Check sheet for the modelled part. Datum: model origin and axes. Units: mm. A direction names the side the tool comes from. Round coordinates to 2 decimals unless told otherwise and drop trailing zeros. Loops run counter-clockwise (first coordinate to the right, second up) from the corner with the lowest first, then second, coordinate; pieces in that order, holes last. Notation, with made-up numbers: (-35.5, 48) - (-23.5, 48) arc R9 cw to (-23.5, 64) - close; hole circle Ø2 at (52, 57). An arc over 180 degrees is marked (long way). Put each result on its own line as item: value.
```python
from build123d import *

# Parameters (mm, degrees)
BOSS_EXTRUDE1_DEPTH = 10
SKETCH2_W           = 5
SKETCH2_H           = 32
BOSS_EXTRUDE2_DEPTH = 18
SKETCH3_W           = 24
SKETCH3_H           = 20
BOSS_EXTRUDE3_DEPTH = 7
CUT_EXTRUDE1_DEPTH  = 56.290143787
BOSS_EXTRUDE4_REACH = 56.194
SKETCH7_R           = 1.7
CUT_EXTRUDE2_DEPTH  = 7
SKETCH6_W           = 8
SKETCH6_H           = 2.8
CUT_EXTRUDE3_DEPTH  = 13.34
SKETCH8_R           = 1.95
CUT_EXTRUDE4_DEPTH  = 55.194244669
FILLET1_R           = 5
FILLET2_R           = 1.25
FILLET3_R           = 6
SKETCH9_W           = 18
SKETCH9_H           = 2.5
BOSS_EXTRUDE5_DEPTH = 4
FILLET4_R           = 1


with BuildPart() as part:
    # Sketch1 → Boss-Extrude1 (new body)
    with BuildSketch(Plane(origin=(0, 0, 0), x_dir=(1, 0, 0), z_dir=(0, 1, 0))):
        Polygon((-17.769938204, -26), (-17.769938204, -20), (-7.769938204, -20), (-7.769938204, 0), (-17.769938204, 0), (-17.769938204, 6), (26.230061796, 6), (26.230061796, 0), (16.230061796, 0), (16.230061796, -20), (26.230061796, -20), (26.230061796, -26), align=None)
    extrude(amount=BOSS_EXTRUDE1_DEPTH)

    # Sketch2 → Boss-Extrude2 (add)
    with BuildSketch(Plane(origin=(0, 10, 0), x_dir=(1, 0, 0), z_dir=(0, 1, 0))):
        with Locations((-5.269938204, -10)):
            Rectangle(SKETCH2_W, SKETCH2_H)
        with Locations((13.730061796, -10)):
            Rectangle(SKETCH2_W, SKETCH2_H)
    extrude(amount=BOSS_EXTRUDE2_DEPTH)

    # Sketch3 → Boss-Extrude3 (add)
    with BuildSketch(Plane(origin=(0, 28, 0), x_dir=(1, 0, 0), z_dir=(0, 1, 0))):
        with Locations((4.230061796, -10)):
            Rectangle(SKETCH3_W, SKETCH3_H)
    extrude(amount=BOSS_EXTRUDE3_DEPTH)

    # Sketch4 → Cut-Extrude1 (cut, through all)
    with BuildSketch(Plane(origin=(16.230061796, 0, 0), x_dir=(0, 0, -1), z_dir=(1, 0, 0))):
        with BuildLine():
            Line((-26, 10), (-26, 35))
            Line((-26, 35), (-18.555107994, 35))
            add(Edge.make_bspline(
                [(-26, 10), (-25.555357091, 18.878891188), (-18.529592831, 25.955762579), (-18.555107994, 35)],
                knots=[0, 0, 0, 0, 1, 1, 1, 1], degree=3))
        make_face()
        with BuildLine():
            Line((6, 10), (6, 35))
            Line((6, 35), (-1.444892006, 35))
            add(Edge.make_bspline(
                [(6, 10), (5.555357091, 18.878891188), (-1.470407169, 25.955762579), (-1.444892006, 35)],
                knots=[0, 0, 0, 0, 1, 1, 1, 1], degree=3))
        make_face()
    extrude(amount=-CUT_EXTRUDE1_DEPTH, mode=Mode.SUBTRACT)

    # Boss-Extrude4: up to this face of the body (flat: up to its plane)
    boss_extrude4_end = Plane(part.part.faces().sort_by_distance((4.230061796, 5, -6))[0])
    # Sketch5 → Boss-Extrude4 (add, up to the picked face)
    with BuildSketch(Plane.XY.offset(26), mode=Mode.PRIVATE) as boss_extrude4_sk1:
        with BuildLine():
            Line((-2.769938204, 10), (11.230061796, 10))
            Line((11.230061796, 10), (11.230061796, 16.5))
            ThreePointArc((11.230061796, 16.5), (11.083615187, 16.853553391), (10.730061796, 17))
            Line((10.730061796, 17), (9.730061796, 17))
            Line((9.730061796, 17), (4.598638866, 11.402084076))
            ThreePointArc((4.598638866, 11.402084076), (4.230061796, 11.239946391), (3.861484726, 11.402084076))
            Line((3.861484726, 11.402084076), (-1.269938204, 17))
            Line((-1.269938204, 17), (-2.269938204, 17))
            ThreePointArc((-2.269938204, 17), (-2.623491594, 16.853553391), (-2.769938204, 16.5))
            Line((-2.769938204, 16.5), (-2.769938204, 10))
        make_face()
    boss_extrude4_tool1 = split(extrude(boss_extrude4_sk1.sketch, amount=-BOSS_EXTRUDE4_REACH, mode=Mode.PRIVATE), bisect_by=boss_extrude4_end, keep=Keep.BOTH, mode=Mode.PRIVATE)
    add(boss_extrude4_tool1.solids().sort_by(Axis((-2.613413, 13.25, 26), (0, 0, -1)))[0])

    # Sketch7 → Cut-Extrude2 (cut)
    with BuildSketch(Plane(origin=(0, 35, 0), x_dir=(1, 0, 0), z_dir=(0, 1, 0))):
        with Locations(Location((4.230061796, -10.360107994, 0), (0, 0, 270))):
            Circle(SKETCH7_R)
    extrude(amount=-CUT_EXTRUDE2_DEPTH, mode=Mode.SUBTRACT)

    # Sketch6 → Cut-Extrude3 (cut)
    with BuildSketch(Plane.XY.offset(20.5)):
        with Locations((4.230061796, 31.5)):
            Rectangle(SKETCH6_W, SKETCH6_H)
    extrude(amount=-CUT_EXTRUDE3_DEPTH, mode=Mode.SUBTRACT)

    # Sketch8 → Cut-Extrude4 (cut, through all)
    with BuildSketch(Plane.XY.offset(26)):
        with Locations((21.230061796, 5)):
            Circle(SKETCH8_R)
        with Locations((-12.769938204, 5)):
            Circle(SKETCH8_R)
    extrude(amount=-CUT_EXTRUDE4_DEPTH, mode=Mode.SUBTRACT)

    # Fillet1
    fillet1_edges = [part.edges().sort_by_distance(p)[0] for p in [
        (-17.769938204, 0, -3),
        (-17.769938204, 10, -3),
        (-17.769938204, 0, 23),
        (-17.769938204, 10, 23),
        (26.230061796, 10, -3),
        (26.230061796, 0, -3),
        (26.230061796, 0, 23),
        (26.230061796, 10, 23),
    ]]
    fillet(fillet1_edges, radius=FILLET1_R - 0.0001)  # a hair under: the kernel refuses the full size

    # Fillet2
    fillet2_edges = [part.edges().sort_by_distance(p)[0] for p in [
        (-7.769938204, 5, 20),
        (-7.769938204, 5, 0),
        (16.230061796, 5, 0),
        (16.230061796, 5, 20),
    ]]
    fillet(fillet2_edges, radius=FILLET2_R)

    # Fillet3
    fillet3_edges = [part.edges().sort_by_distance(p)[0] for p in [
        (16.230061796, 35, 10),
        (-7.769938204, 35, 10),
    ]]
    fillet(fillet3_edges, radius=FILLET3_R)

    # Sketch9 → Boss-Extrude5 (add)
    with BuildSketch(Plane.XZ):
        with Locations((4.230061796, 24.75)):
            Rectangle(SKETCH9_W, SKETCH9_H)
    extrude(amount=BOSS_EXTRUDE5_DEPTH)

    # Fillet4
    fillet4_edges = [part.edges().sort_by_distance(p)[0] for p in [
        (4.230061796, 0, 23.5),
    ]]
    fillet(fillet4_edges, radius=FILLET4_R)


solid = part.part
```
Item 1: Section check C-C on y = 8.5. Enter the section's corners in (x, z), then the cut area to 3 significant figures.
Filled sheet:
outline: (-16.34, -6) - (24.8, -6) - (24.8, 0) - (17.48, 0) arc R1.25 cw to (16.23, 1.25) - (16.23, 18.75) arc R1.25 cw to (17.48, 20) - (24.8, 20) - (24.8, 26) - (-16.34, 26) - (-16.34, 20) - (-9.02, 20) arc R1.25 cw to (-7.77, 18.75) - (-7.77, 1.25) arc R1.25 cw to (-9.02, 0) - (-16.34, 0) - close
area: 975 mm²
Item 2: Section check A-A on z = 14.5. Enter the section's corners in (x, y), then the cut area to 3 significant figures.
Filled sheet:
outline: (-7.77, 0) - (16.23, 0) - (16.23, 29) arc R6 ccw to (10.23, 35) - (-1.77, 35) arc R6 ccw to (-7.77, 29) - close; hole (-2.77, 16.5) arc R0.5 cw to (-2.27, 17) - (-1.27, 17) - (3.86, 11.4) arc R0.5 ccw to (4.6, 11.4) - (9.73, 17) - (10.73, 17) arc R0.5 cw to (11.23, 16.5) - (11.23, 28) - (-2.77, 28) - close; hole (0.23, 30.1) - (8.23, 30.1) - (8.23, 32.9) - (0.23, 32.9) - close
area: 615 mm²
Item 3: Release check for a two-part mould opening along Z. For faces 6 (the flat face through (19, 10, -3)), 7 (the flat face through (22, 3, 0)), 8 (the flat face through (4, 6, -6)) record: +Z half, -Z half, draft (parallel to the pull), parting line (faces both ways), or undercut.
Filled sheet:
face 6: draft
face 7: undercut
face 8: -Z half
Item 4: Section check B-B on x = -12. Enter the section's corners in (y, z).
Filled sheet:
outline: (0, -6) - (3.21, -6) - (3.21, 0) - (0, 0) - close; (0, 20) - (3.21, 20) - (3.21, 26) - (0, 26) - close; (6.79, -6) - (10, -6) - (10, 0) - (6.79, 0) - close; (6.79, 20) - (10, 20) - (10, 26) - (6.79, 26) - close
Item 5: Thickness scan on line 1 (Z direction, x = 19, y = 5); line 2 (Y direction, x = 3, z = 17.5); line 3 (Y direction, x = 8, z = 8.5). Record the ranges inside material, lowest first. Write a range as from..to.
Filled sheet:
line 1: -6..0, 20..26
line 2: 0..12.34, 28..30.1, 32.9..35
line 3: 0..15.11, 28..30.1, 32.9..35
Item 6: Go/stop test with flat-tipped pins: pin 1 (1.5 mm diameter, centred on y = 23.5, z = 13, fed in from -X); pin 2 (1.5 mm diameter, centred on x = 17.5, y = 30, fed in from -Z); pin 3 (9.5 mm diameter, centred on x = 0, z = 7.5, fed in from -Y); pin 4 (5 mm diameter, centred on y = 13, z = 22, fed in from +X). Record where each tip stops, or that it passes through.
Filled sheet:
pin 1: x = -7.77
pin 2: through
pin 3: y = 0
pin 4: x = 16.23
Item 7: Tool access check on faces 1 (the flat face through (0.23, 31, 13)), 2 (the flat face through (7.2, 14.24, 10.22)), 3 (the flat face through (4, -2, 23.5)), 4 (the flat face through (-7.77, 14, 10)), 5 (the flat face through (11.23, 14.6, -5.6)). Record the directions out of +Z, -Z, +X, -X, +Y, -Y that give a thin tool (end or side, any length) a straight path to the whole face; none if there is none.
Filled sheet:
face 1: +Z
face 2: +Z, -Z
face 3: -Z, +X, -X, -Y
face 4: -X, +Y
face 5: -Z, +X, +Y
